```python
from build123d import *

# Parameters (mm, degrees)
SKETCH1_W           = 442
SKETCH1_H           = 80
BOSS_EXTRUDE1_DEPTH = 2.5
SKETCH7_W           = 5
SKETCH7_H           = 25
BOSS_EXTRUDE2_DEPTH = 5
SKETCH8_W           = 5
SKETCH8_H           = 15
CUT_EXTRUDE6_DEPTH  = 4
SKETCH4_W           = 5.2
SKETCH4_H           = 40
CUT_EXTRUDE7_DEPTH  = 10
SKETCH10_W          = 20.2
SKETCH10_H          = 10
CUT_EXTRUDE8_DEPTH  = 300
SKETCH11_R          = 5
CUT_EXTRUDE9_DEPTH  = 10


with BuildPart() as part:
    # Sketch1 → Boss-Extrude1 (new, symmetric)
    with BuildSketch(Plane.XY):
        with Locations((0, 40)):
            Rectangle(SKETCH1_W, SKETCH1_H)
    extrude(amount=BOSS_EXTRUDE1_DEPTH, both=True)

    # Sketch7 → Boss-Extrude2 (add)
    with BuildSketch(Plane(origin=(221, 0, 0), x_dir=(0, 0, -1), z_dir=(1, 0, 0))):
        with Locations((0, 62.5)):
            Rectangle(SKETCH7_W, SKETCH7_H)
        with Locations((0, 27.4)):
            Rectangle(SKETCH7_W, SKETCH7_H)
    boss_extrude2 = extrude(amount=BOSS_EXTRUDE2_DEPTH)

    # Sketch8 → Cut-Extrude6 (cut)
    with BuildSketch(Plane(origin=(226, 0, 0), x_dir=(0, 0, -1), z_dir=(1, 0, 0))):
        with Locations((0, 62.5)):
            Rectangle(SKETCH8_W, SKETCH8_H)
        with Locations((0, 27.4)):
            Rectangle(SKETCH8_W, SKETCH8_H)
    cut_extrude6 = extrude(amount=-CUT_EXTRUDE6_DEPTH, mode=Mode.SUBTRACT)

    # Mirror8: Boss-Extrude2, Cut-Extrude6 across plane
    add(boss_extrude2.mirror(Plane(origin=(0, 0, 0), x_dir=(0, 0, 1), z_dir=(1, 0, 0))))
    add(cut_extrude6.mirror(Plane(origin=(0, 0, 0), x_dir=(0, 0, 1), z_dir=(1, 0, 0))), mode=Mode.SUBTRACT)

    # Sketch4 → Cut-Extrude7 (cut)
    with BuildSketch(Plane.XY.offset(2.5)):
        with Locations((0, 20)):
            Rectangle(SKETCH4_W, SKETCH4_H)
    extrude(amount=-CUT_EXTRUDE7_DEPTH, mode=Mode.SUBTRACT)

    # Sketch10 → Cut-Extrude8 (cut)
    with BuildSketch(Plane(origin=(0, -565.456150304, -2.5), x_dir=(-1, 0, 0), z_dir=(0, 0, -1))):
        with Locations((27.5, 585.456150304)):
            Rectangle(SKETCH10_W, SKETCH10_H)
    cut_extrude8 = extrude(amount=-CUT_EXTRUDE8_DEPTH, mode=Mode.SUBTRACT)

    # Mirror9: Cut-Extrude8 across plane
    add(cut_extrude8.mirror(Plane(origin=(0, 0, 0), x_dir=(0, 0, 1), z_dir=(1, 0, 0))), mode=Mode.SUBTRACT)

    # Sketch11 → Cut-Extrude9 (cut)
    with BuildSketch(Plane(origin=(0, 0, -2.5), x_dir=(-1, 0, 0), z_dir=(0, 0, -1))):
        with Locations((-114.385224348, 39.9)):
            Circle(SKETCH11_R)
        with Locations(Location((114.385224348, 39.9, 0), (0, 0, 180))):
            Circle(SKETCH11_R)
    extrude(amount=-CUT_EXTRUDE9_DEPTH, mode=Mode.SUBTRACT)


solid = part.part
```
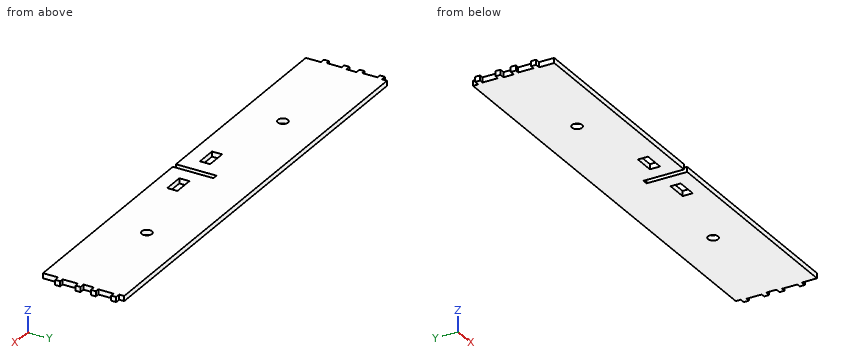
Model file for the job. Use its own axes, mm. Round coordinates to 2 decimals unless told otherwise and drop trailing zeros. Use CSV: the item, a comma, the result in double quotes.
Item 1: Probe probe 1 along X at (y, z) = (22.5, -0.45); probe 2 along X at (y, z) = (30, -1.35); probe 3 along Y at (x, z) = (-22.5, -1.2). List the from-to ranges inside material, lowest first.
Worked answers:
probe 1,"-222 to -37.6, -17.4 to -2.6, 2.6 to 17.4, 37.6 to 222"
probe 2,"-222 to -2.6, 2.6 to 222"
probe 3,"0 to 15, 25 to 80"
Item 2: Saw through at A-A (z = 0.5). State how many separate pieces and enclosed holes the cut face has, plus the area to 3 significant figures.
Worked answers:
separate pieces,"1"
enclosed holes,"4"
area,"34,900 mm²"
Item 3: Pin check, flat tips, straight feed: pin 1 (1.5 mm diameter, centred on y = 5.5, z = 0, fed in from -X); pin 2 (1.5 mm diameter, centred on x = 223.5, z = -0.5, fed in from +Y); pin 3 (9 mm diameter, centred on x = 114.39, y = 39.9, fed in from -Z); pin 4 (1.5 mm diameter, centred on x = 223.5, z = 0.5, fed in from -Y). Stop position of each tip, or through.
Worked answers:
pin 1,"x = -221"
pin 2,"y = 75"
pin 3,"through"
pin 4,"y = 14.9"
